Study the drawing (mm; zero at the part's minimum x, y, z) and answer. Give positions to 0.01 mm unless a question says otherwise; leave off trailing zeros. Loops run counter-clockwise (first coordinate to the right, second up) from the corner with the lowest first, then second, coordinate; pieces in that order, holes last. Notation, with made-up numbers: M 18.5,-32.75 L 35.5,-32.75 A25 cw 35.5,-20.75 Z; hole C 86,-30 d10. An arc over 180 degrees is marked long. Return JSON: item names as keys, results as strings.
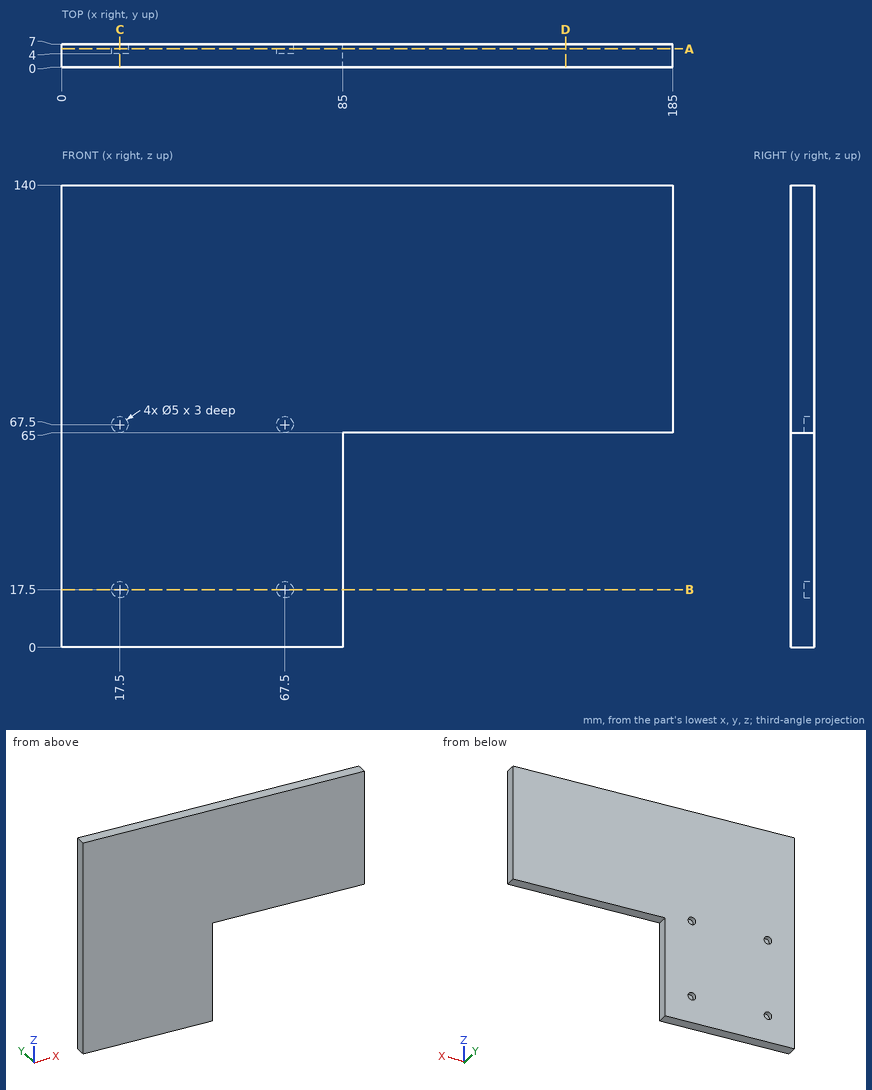
(1) The part is cut by section A-A (y = 5.5). Determine the outline of the cut face in (x, z), and give its area (3 significant figures).
Values follow:
{"outline": "M 0,0 L 85,0 L 85,65 L 185,65 L 185,140 L 0,140 Z; hole C 17.5,17.5 d5; hole C 17.5,67.5 d5; hole C 67.5,17.5 d5; hole C 67.5,67.5 d5", "area": "19,300 mm²"}
(2) The part is cut by section B-B (z = 17.5). Determine the outline of the cut face in (x, y), and give its area (3 significant figures).
Values follow:
{"outline": "M 0,0 L 85,0 L 85,7 L 70,7 L 70,4 L 65,4 L 65,7 L 20,7 L 20,4 L 15,4 L 15,7 L 0,7 Z", "area": "565 mm²"}
(3) The part is cut by section D-D (x = 152.5). Determine the outline of the cut face in (y, z).
Values follow:
{"outline": "M 0,65 L 7,65 L 7,140 L 0,140 Z"}
(4) Straight lines are drawn through the part: line 1 along Z through (x, y) = (17.5, 5.75); line 2 along X through (y, z) = (4.95, 67.5); line 3 along X through (y, z) = (1, 13). For each, find the intervals that lie inside material, in ascending order.
Values follow:
{"line 1": "0 to 15, 20 to 65, 70 to 140", "line 2": "0 to 15, 20 to 65, 70 to 185", "line 3": "0 to 85"}
(5) Given pin 1 (1 mm diameter, centred on x = 166, y = 3.5, fed in from -Z); pin 2 (4.5 mm diameter, centred on x = 67.5, z = 67.5, fed in from +Y); pin 3 (2 mm diameter, centred on y = 5, z = 56.5, fed in from +X), each flat-ended and moving along its own axis, determine where each tip first touches the part or whether it passes through.
Values follow:
{"pin 1": "z = 65", "pin 2": "y = 4", "pin 3": "x = 85"}
(6) The part is cut by section C-C (x = 17.5). Determine the outline of the cut face in (y, z), and give its area (3 significant figures).
Values follow:
{"outline": "M 0,0 L 7,0 L 7,15 L 4,15 L 4,20 L 7,20 L 7,65 L 4,65 L 4,70 L 7,70 L 7,140 L 0,140 Z", "area": "950 mm²"}
